```python
from build123d import *

# Parameters (mm, degrees)
F1_DEPTH = 28.448
F2_W     = 35.3105356917
F2_H     = 30.2078574896
F3_DEPTH = 73.152


# Not quite as in the source:
# - a feature names something its author has since deleted; it is built from what else it names


with BuildPart() as f1:
    # F0 (on Front) → F1 (new body)
    with BuildSketch(Plane.XZ):
        Polygon((21.7242818326, 32.0553742349), (-39.2557755113, 32.1793556213), (-39.2557755113, -16.2723716348), (21.7242818326, -16.2723716348), align=None)
    extrude(amount=F1_DEPTH)

    # F2 (on Front) → F3 (join)
    with BuildSketch(Plane.XZ):
        with Locations((-8.470446337, -1.2246426195)):
            Rectangle(F2_W, F2_H)
    extrude(amount=F3_DEPTH)


solid = f1.part
```
Design review of the part built by this model. Coordinates are the model's own, in mm. Coordinates: 2 decimals unless noted, no trailing zeros. Order: outer loops, then holes, each group sorted by start corner. A loop starts at its lowest first (then second) coordinate and runs counter-clockwise, first axis right, second up.
1) Take a section at C-C, the plane y = -66.5. Give the boundary of the cut face in (x, z).
2) Take a section at A-A, the plane z = 6.5. Give the boundary of the cut face in (x, y).
3) Wall thickness on line 1 along X through (y, z) = (-39.5, -14); line 2 along Y through (x, z) = (-1, 19.5); line 3 along Z through (x, y) = (13.5, -26): over which ranges is each line inside the solid? List them lowest first.
4) Take a section at B-B, the plane x = -19. Give the boundary of the cut face in (y, z), and give its area (3 significant figures).
5) Clearance check with flat-ended pins moving along their axes: pin 1 (12 mm diameter, centred on x = 5.5, z = 14, fed in from -Y); pin 2 (10.5 mm diameter, centred on x = -5, y = -49, fed in from +Z); pin 3 (6 mm diameter, centred on y = -34, z = 9.5, fed in from -X); pin 4 (4 mm diameter, centred on x = 18.5, y = -20, fed in from -Z). State where each tip first meets the part, or that it passes through.
6) Take a section at D-D, the plane x = -9. Give the boundary of the cut face in (y, z).
Returned:
1. outline: (-26.13, -16.33) - (9.18, -16.33) - (9.18, 13.88) - (-26.13, 13.88) - close
2. outline: (-39.26, -28.45) - (-26.13, -28.45) - (-26.13, -73.15) - (9.18, -73.15) - (9.18, -28.45) - (21.72, -28.45) - (21.72, 0) - (-39.26, 0) - close
3. line 1: x = -26.13 to 9.18
3. line 2: y = -28.45 to 0
3. line 3: z = -16.27 to 32.07
4. outline: (-73.15, -16.33) - (0, -16.33) - (0, 32.14) - (-28.45, 32.14) - (-28.45, 13.88) - (-73.15, 13.88) - close
4. area: 2,730 mm2
5. pin 1: stops at y = -73.15
5. pin 2: stops at z = 13.88
5. pin 3: stops at x = -26.13
5. pin 4: stops at z = -16.27
6. outline: (-73.15, -16.33) - (0, -16.33) - (0, 32.12) - (-28.45, 32.12) - (-28.45, 13.88) - (-73.15, 13.88) - close
